Build history of the part. All positions in model axes, mm. Face numbers are marked on the shaded views. A direction names the side the tool comes from. Round coordinates to 2 decimals unless told otherwise and drop trailing zeros. Write each loop counter-clockwise with the first axis right and the second up, starting at its lowest first coordinate (ties: lowest second). Pieces come first, ordered by that corner, then holes.
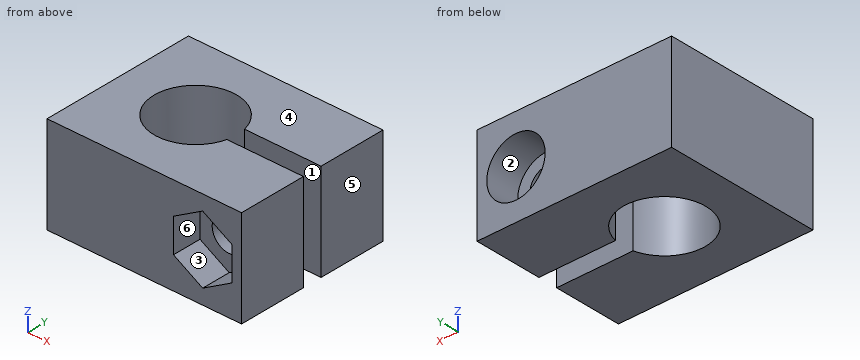
from build123d import *

# Parameters (mm, degrees)
PAD_DEPTH       = 10
SKETCH001_R     = 1.75
POCKET_DEPTH    = 16
SKETCH002_R     = 3
POCKET001_DEPTH = 3.5
POCKET002_DEPTH = 3


with BuildPart() as part:
    # Sketch → Pad (new body)
    with BuildSketch(Plane.XY):
        with BuildLine():
            Line((0, 0), (0, 16))
            Line((0, 16), (20, 16))
            Line((20, 16), (20, 9))
            Line((20, 9), (12.130678, 9))
            ThreePointArc((12.130678, 9), (3.75, 8), (12.130678, 7))
            Line((12.130678, 7), (20, 7))
            Line((20, 7), (20, 0))
            Line((20, 0), (0, 0))
        make_face()
    extrude(amount=PAD_DEPTH)

    # Sketch001 → Pocket (cut)
    with BuildSketch(Plane(origin=(0, 16, 0), x_dir=(-1, 0, 0), z_dir=(0, 1, 0))):
        with Locations((-16, 4.999996)):
            Circle(SKETCH001_R)
    extrude(amount=-POCKET_DEPTH, mode=Mode.SUBTRACT)

    # Sketch002 → Pocket001 (cut)
    with BuildSketch(Plane(origin=(0, 16, 0), x_dir=(-1, 0, 0), z_dir=(0, 1, 0))):
        with Locations((-16, 5)):
            Circle(SKETCH002_R)
    extrude(amount=-POCKET001_DEPTH, mode=Mode.SUBTRACT)

    # Sketch003 → Pocket002 (cut)
    with BuildSketch(Plane.XZ):
        Polygon((15.999999, 8.461405), (13, 6.729354), (13, 3.265252), (16, 1.533202), (19, 3.265253), (19, 6.729355), align=None)
    extrude(amount=-POCKET002_DEPTH, mode=Mode.SUBTRACT)


solid = part.part
1) Slice it at B-B (z = 1). Write the cut outline in (x, y).
Results:
outline: (0, 0) - (20, 0) - (20, 7) - (12.13, 7) arc R4.25 cw (long way) to (12.13, 9) - (20, 9) - (20, 16) - (0, 16) - close
2) Slice it at A-A (x = 8). Write the cut outline in (y, z), plus the area to 3 significant figures.
Results:
outline: (0, 0) - (3.75, 0) - (3.75, 10) - (0, 10) - close; (12.25, 0) - (16, 0) - (16, 10) - (12.25, 10) - close
area: 75.0 mm2
3) Which spindle directions (+Z, -Z, +X, -X, +Y, -Y) get a long thin tool onto all of the face, cutting with end or side? Do the marked faces 1, 2 and 3. Say none if no direction does.
Results:
face 1: +Z, -Z, +X
face 2: +Y
face 3: -Y
4) Mould opens along Z. For the marked faces 4, 5 and 6 say: released by +Z, released by -Z, zero draft, split by the parting line, or undercut.
Results:
face 4: released by +Z
face 5: zero draft
face 6: undercut
5) Slice it at C-C (y = 14). Write the cut outline in (x, z).
Results:
outline: (0, 0) - (20, 0) - (20, 10) - (0, 10) - close; hole circle Ø6 at (16, 5)
6) Slice it at D-D (x = 4). Write the cut outline in (y, z).
Results:
outline: (0, 0) - (6.56, 0) - (6.56, 10) - (0, 10) - close; (9.44, 0) - (16, 0) - (16, 10) - (9.44, 10) - close
7) Pin check, flat tips, straight feed: pin 1 Ø1.5 at (x, z) = (15.5, 6.5) entering from -Y; pin 2 Ø3 at (x, z) = (17, 5) entering from +Y; pin 3 Ø1.5 at (x, y) = (7.5, 10.5) entering from -Z. Stop position of each tip, or through.
Results:
pin 1: stops at y = 3
pin 2: stops at y = 12.5
pin 3: passes through
8) Wall check: L1, parallel to Z at x = 15.75, y = 4.75; L2, parallel to Y at x = 15.5, z = 0.5; L3, parallel to Y at x = 14, z = 6.5. Give the ranges that are in metal, low to high.
Results:
L1: z = 0 to 3.27, 6.73 to 10
L2: y = 0 to 7, 9 to 16
L3: y = 3 to 7, 9 to 12.5
